Source: CAD feature listing. Evaluate the final solid. Frame: model axes, mm. A direction names the side the tool comes from. Give positions to 0.01 mm unless a question says otherwise; leave off trailing zeros. Write each loop counter-clockwise with the first axis right and the second up, starting at its lowest first coordinate (ties: lowest second). Pieces come first, ordered by that corner, then holes.
Autodesk Inventor part; units mm, degrees
ref_plane "Work Plane1" through (0, 8, 0) normal (0, 1, 0) x (1, 0, 0)
ref_plane "Work Plane2" through (0, -12.4, 0) normal (0, -1, 0) x (1, 0, 0)
ref_plane "YZ Plane" through (0, 0, 0) normal (1, 0, 0) x (0, 1, 0)
sketch "Sketch1" plane through (0, 0, 0) normal (0, 1, 0) x (-1, 0, 0)
  line L0 (0, 5.7735) -> (5, 2.8868)
  line L1 (5, 2.8868) -> (5, -2.8868)
  line L2 (5, -2.8868) -> (0, -5.7735)
  line L3 (0, -5.7735) -> (-5, -2.8868)
  line L4 (-5, -2.8868) -> (-5, 2.8868)
  line L5 (-5, 2.8868) -> (0, 5.7735)
  point P0 (0, 0)
  dimension "d24" = 10
extrude "Extrusion1" add sketch "Sketch1" along normal blind 2
sketch "Sketch2" plane through (0, 2, 0) normal (0, 1, 0) x (1, 0, 0)
  circle A0 centre (0, 0) radius 3.5
  dimension "d2" = 7
ref_plane "Work Plane1" through (0, 8, 0) normal (0, 1, 0) x (1, 0, 0)
sketch "Sketch3" plane through (0, 8, 0) normal (0, 1, 0) x (1, 0, 0)
  circle A0 centre (0, 0) radius 1.75
  dimension "d4" = 3.5
loft "Loft1" add profiles "Sketch2", "Sketch3"
sketch "Sketch4" plane through (0, 0, 0) normal (0, -1, 0) x (1, 0, 0)
  circle A0 centre (0, 0) radius 4
  dimension "d9" = 8
extrude "Extrusion2" add sketch "Sketch4" along normal blind 10.4
thread "Thread1"
sketch "Sketch5" plane through (0, 8, 0) normal (0, 1, 0) x (1, 0, 0)
  circle A0 centre (0, 0) radius 1
  dimension "d14" = 2
ref_plane "Work Plane2" through (0, -12.4, 0) normal (0, -1, 0) x (1, 0, 0)
sketch "Sketch6" plane through (0, -12.4, 0) normal (0, -1, 0) x (1, 0, 0)
  circle A0 centre (0, 0) radius 2.25
  dimension "d16" = 4.5
sketch "Sketch7" plane through (0, -10.4, 0) normal (0, -1, 0) x (1, 0, 0)
  circle A0 centre (0, 0) radius 3.25
  dimension "d17" = 6.5
loft "Loft2" add profiles "Sketch7", "Sketch6"
extrude "Extrusion3" cut sketch "Sketch5" against normal up to surface (20.4 mm away)
properties part number "ZKE-Term-Solid"
1. Access query for faces 4 (the flat face through (-2, -10.4, 3)), 5 (the flat face through (-5, 1, 0)). Directions: +Z, -Z, +X, -X, +Y, -Y. A direction counts if a zero-diameter tool reaches every point of the face in a straight line with its end or side. Return the directions, or none.
2. Section query D-D (y = 6.5). Return loops of the section in (x, z) (1 decimal).
3. Section query A-A (y = 1). Return loops of the section in (x, z), plus the area to 3 significant figures.
4. Section query B-B (z = -4.25). Return loops of the section in (x, y), plus the area to 3 significant figures.
5. Pin query (flat end, axial travel): P1, Ø2, axis at y = -7.5, z = -2.5, coming from the +X side; P2, Ø2, axis at y = -3.5, z = -1.5, coming from the -X side. Return the tip coordinate at first contact, or that it passes through.
6. Section query C-C (y = -6.75). Return loops of the section in (x, z), plus the area to 3 significant figures.
7. Pull-direction query (X, two-part tool) for faces 1 (the conical face through (2.33, 5.625, 0.734)), 2 (the cylindrical face through (0, -2, 1)), 3 (the flat face through (0, 2, -4)); classes: pulls with the +X half, pulls with the -X half, needs draft (parallel to the pull), parting line crosses it, or undercut.
8. Line query: probe 1 along Z at (x, y) = (0, -3); probe 2 along Y at (x, z) = (1.25, -3.5); probe 3 along Z at (x, y) = (0.75, -10). Output: solid intervals per line, ascending.
The answers:
1. face 4: -Y
1. face 5: +Z, -Z, -X, +Y, -Y
2. outline: circle Ø4.4 at (0, 0); hole circle Ø2 at (0, 0)
3. outline: (-5, -2.89) - (0, -5.77) - (5, -2.89) - (5, 2.89) - (0, 5.77) - (-5, 2.89) - close; hole circle Ø2 at (0, 0)
3. area: 83.5 mm2
4. outline: (-2.64, 0) - (2.64, 0) - (2.64, 2) - (-2.64, 2) - close
4. area: 10.6 mm2
5. P1: stops at x = 3.71
5. P2: stops at x = -3.97
6. outline: circle Ø8 at (0, 0); hole circle Ø2 at (0, 0)
6. area: 47.1 mm2
7. face 1: parting line crosses it
7. face 2: undercut
7. face 3: needs draft
8. probe 1: z = -4 to -1, 1 to 4
8. probe 2: y = -10.4 to 2
8. probe 3: z = -3.93 to -0.66, 0.66 to 3.93
